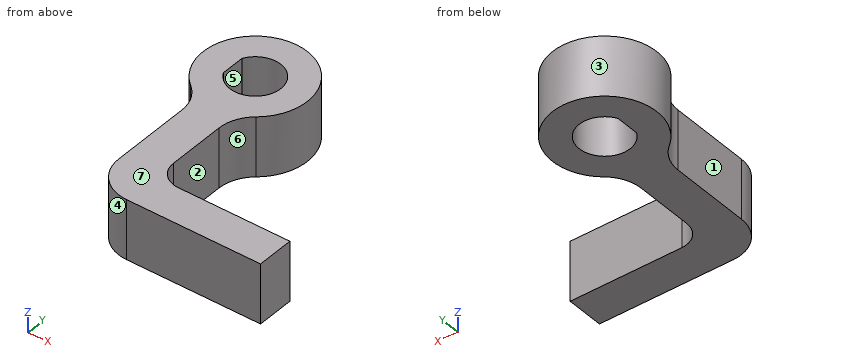
```python
from build123d import *

# Parameters (mm, degrees)
BOSS_EXTRUDE1_DEPTH = 4


with BuildPart() as part:
    # Sketch1 → Boss-Extrude1 (new, symmetric)
    with BuildSketch(Plane.XY):
        with BuildLine():
            Line((-2.5, -9.367496998), (-2.5, -20.15))
            ThreePointArc((-2.5, -20.15), (-1.035533906, -23.685533906), (2.5, -25.15))
            Line((2.5, -25.15), (20.5, -25.15))
            Line((20.5, -25.15), (20.5, -20.15))
            Line((20.5, -20.15), (5.5, -20.15))
            ThreePointArc((5.5, -20.15), (3.378679656, -19.271320344), (2.5, -17.15))
            Line((2.5, -17.15), (2.5, -9.367496998))
            ThreePointArc((2.5, -9.367496998), (2.993060906, -7.202433488), (4.375, -5.464373249))
            ThreePointArc((4.375, -5.464373249), (0, 7), (-4.375, -5.464373249))
            ThreePointArc((-4.375, -5.464373249), (-2.993060906, -7.202433488), (-2.5, -9.367496998))
        make_face()
        with BuildLine():
            Line((-3.04, 1.577664413), (-3.04, -1.577664413))
            ThreePointArc((-3.04, -1.577664413), (3.425, 0), (-3.04, 1.577664413))
        make_face(mode=Mode.SUBTRACT)
    extrude(amount=BOSS_EXTRUDE1_DEPTH, both=True)


solid = part.part
```
The listing builds one solid part. Answer for the finished solid, in the listing's coordinates (mm). Face numbers are marked on the shaded views. A direction names the side the tool comes from. Round coordinates to 2 decimals unless told otherwise and drop trailing zeros. Order: outer loops, then holes, each group sorted by start corner. A loop starts at its lowest first (then second) coordinate and runs counter-clockwise, first axis right, second up. Notation, with made-up numbers: (5, 36) -> (33, 36) arc R21 ccw to (33, 41) -> close; hole circle Ø5 at (3, -3.75). An arc over 180 degrees is marked (long way). Answer as CSV lines item,"result".
Q1. A cutting plane is placed at C-C on x = -1.5. Determine the outline of the cut face in (y, z), plus the area to 3 significant figures.
Computed values:
outline,"(-23.15, -4) -> (-3.08, -4) -> (-3.08, 4) -> (-23.15, 4) -> close; (3.08, -4) -> (6.84, -4) -> (6.84, 4) -> (3.08, 4) -> close"
area,"191 mm^2"
Q2. For a pull along Y with two mould halves and no side action, classify the marked faces 4, 5, 6 and 7 as +Y half, -Y half, draft (parallel to the pull), parting line (faces both ways), or undercut.
Computed values:
face 4,"-Y half"
face 5,"undercut"
face 6,"undercut"
face 7,"draft"
Q3. A cutting plane is placed at A-A on y = 0. Determine the outline of the cut face in (x, z) (3 decimals).
Computed values:
outline,"(-7, -4) -> (-3.04, -4) -> (-3.04, 4) -> (-7, 4) -> close; (3.425, -4) -> (7, -4) -> (7, 4) -> (3.425, 4) -> close"
Q4. Given pin 1 (2.5 mm diameter, centred on y = -16.5, z = -0.5, fed in from -X); pin 2 (8 mm diameter, centred on x = 0, y = 0, fed in from +Z); pin 3 (2 mm diameter, centred on x = 13, z = -2.5, fed in from +Y); pin 4 (3.5 mm diameter, centred on y = 0.5, z = -1, fed in from +X), each flat-ended and moving along its own axis, determine where each tip first touches the part or whether it passes through.
Computed values:
pin 1,"stops at x = -2.5"
pin 2,"stops at z = 4"
pin 3,"stops at y = -20.15"
pin 4,"stops at x = 7"
Q5. Which of the six approach directions +Z, -Z, +X, -X, +Y, -Y give full straight-line access (tool end or side, diameter ignored) to the marked faces 1, 2 and 3?
Computed values:
face 1,"+Z, -Z, -X, -Y"
face 2,"+Z, -Z, +X"
face 3,"+Z, -Z"
Q6. Consider line 1 (Y direction, x = 9.5, z = -1.5); line 2 (Y direction, x = 3, z = -0.5); line 3 (Y direction, x = 0, z = -0.25) (3 decimals). Determine where each line is inside the solid, lowest interval first. Write a range as from..to.
Computed values:
line 1,"y = -25.15..-20.15"
line 2,"y = -25.15..-18.81, -7.19..-1.65, 1.65..6.32"
line 3,"y = -24.48..-3.425, 3.425..7"
Q7. A cutting plane is placed at D-D on x = 9.5. Determine the outline of the cut face in (y, z), plus the area to 3 significant figures.
Computed values:
outline,"(-25.15, -4) -> (-20.15, -4) -> (-20.15, 4) -> (-25.15, 4) -> close"
area,"40.0 mm^2"
